Input: part model. Units: mm. Frame: model coordinates. A direction names the side the tool comes from. Give positions to 0.01 mm unless a question says otherwise; leave off trailing zeros. Order: outer loops, then holes, each group sorted by start corner. A loop starts at its lowest first (then second) coordinate and runs counter-clockwise, first axis right, second up. Notation, with made-up numbers: M 56,38 L 83,38 A7 cw 83,51 Z; hole C -19.5,74 d7. An arc over 180 degrees is marked long. Use a Markdown table: item, result.
from build123d import *

# Parameters (mm, degrees)
SKETCH_R     = 6
PAD_DEPTH    = 2
SKETCH001_R  = 5
PAD001_DEPTH = 2
SKETCH002_R  = 6
PAD002_DEPTH = 2
SKETCH003_R  = 2.5
POCKET_DEPTH = 6.001


with BuildPart() as part:
    # Sketch → Pad (new body)
    with BuildSketch(Plane.XY):
        Circle(SKETCH_R)
    extrude(amount=PAD_DEPTH)

    # Sketch001 (on Face3 of Pad) → Pad001 (join)
    with BuildSketch(Plane.XY.offset(2)):
        Circle(SKETCH001_R)
    extrude(amount=PAD001_DEPTH)

    # Sketch002 (on Face5 of Pad001) → Pad002 (join)
    with BuildSketch(Plane.XY.offset(4)):
        Circle(SKETCH002_R)
    extrude(amount=PAD002_DEPTH)

    # Sketch003 (on Face3 of Pad002) → Pocket (cut, through all)
    with BuildSketch(Plane.XY.offset(6)):
        Circle(SKETCH003_R)
    extrude(amount=-POCKET_DEPTH, mode=Mode.SUBTRACT)


solid = part.part
1) Cut plane C-C on z = 1. Return loops of the section in (x, y), and give its area (3 significant figures).
Response values:
| item | result |
|---|---|
| outline | C 0,0 d12; hole C 0,0 d5 |
| area | 93.5 mm² |
2) First-contact query: pin 1 Ø2 at (y, z) = (-3, 5.5) entering from +X; pin 2 Ø1 at (x, z) = (-1.5, 4.5) entering from +Y; pin 3 Ø3.5 at (x, y) = (-3, -2.5) entering from -Z. Flat tips, straight axial feed; report the tip coordinate or a pass-through.
Response values:
| item | result |
|---|---|
| pin 1 | stops at x = 5.66 |
| pin 2 | stops at y = 5.92 |
| pin 3 | stops at z = 0 |
3) Reachability of faces 1 (the face through (-1.08, -4.88, 2.99)), 2 (the face through (3, 0, 6)) from +Z, -Z, +X, -X, +Y, -Y: full face, straight path, thin tool, end or side. Return the list, or none.
Response values:
| item | result |
|---|---|
| face 1 | none |
| face 2 | +Z, +X, -X, +Y, -Y |
4) Mould query, pull axis X, two halves, no side actions, for faces 3 (the face through (-6, 0, 5)), 4 (the face through (-0.54, -2.44, 3.04)), 5 (the face through (3, 0, 0)). Classes: released by +X, released by -X, zero draft, split by the parting line, or undercut.
Response values:
| item | result |
|---|---|
| face 3 | split by the parting line |
| face 4 | undercut |
| face 5 | zero draft |
5) Material intervals for line 1 (Y direction, x = 0, z = 2.6); line 2 (Z direction, x = 3, y = 4.5); line 3 (X direction, y = -1, z = 0.95), sorted ascending. Write a range as from..to.
Response values:
| item | result |
|---|---|
| line 1 | y = -5..-2.5, 2.5..5 |
| line 2 | z = 0..2, 4..6 |
| line 3 | x = -5.92..-2.29, 2.29..5.92 |
6) Cut plane A-A on y = 0. Return loops of the section in (x, z), and give its area (3 significant figures).
Response values:
| item | result |
|---|---|
| outline | M -6,0 L -2.5,0 L -2.5,6 L -6,6 L -6,4 L -5,4 L -5,2 L -6,2 Z; M 2.5,0 L 6,0 L 6,2 L 5,2 L 5,4 L 6,4 L 6,6 L 2.5,6 Z |
| area | 38.0 mm² |
7) Cut plane D-D on y = 4.25. Return loops of the section in (x, z).
Response values:
| item | result |
|---|---|
| outline | M -4.24,0 L 4.24,0 L 4.24,2 L 2.63,2 L 2.63,4 L 4.24,4 L 4.24,6 L -4.24,6 L -4.24,4 L -2.63,4 L -2.63,2 L -4.24,2 Z |
